Work out the finished part from the listing and answer in its coordinate system (mm). Round coordinates to 2 decimals unless told otherwise and drop trailing zeros. Order: outer loops, then holes, each group sorted by start corner. A loop starts at its lowest first (then second) coordinate and runs counter-clockwise, first axis right, second up. Notation, with made-up numbers: (42, 48) -> (46, 48) arc R16 ccw to (46, 72) -> close; hole circle Ø9 at (1, 41.25). An arc over 180 degrees is marked (long way). Use one line per item in the form item = value.
```python
from build123d import *

# Parameters (mm, degrees)
SKETCH_1_R          = 1.75
EXTRUDE_1_DEPTH     = 2
SKETCH_3_R          = 1.5
CUT_EXTRUDE_1_DEPTH = 10


with BuildPart() as part:
    # 草图1 → 凸台-拉伸1 (new body)
    with BuildSketch(Plane(origin=(0, 0, 0), x_dir=(1, 0, 0), z_dir=(0, 1, 0))):
        with BuildLine():
            Line((-44.248197972, 34.748679798), (44.751802028, 34.748679798))
            ThreePointArc((44.751802028, 34.748679798), (46.16601559, 34.16289336), (46.751802028, 32.748679798))
            Line((46.751802028, 32.748679798), (46.751802028, -32.251320202))
            ThreePointArc((46.751802028, -32.251320202), (46.16601559, -33.665533764), (44.751802028, -34.251320202))
            Line((44.751802028, -34.251320202), (-45.248197972, -34.251320202))
            ThreePointArc((-45.248197972, -34.251320202), (-46.662411535, -33.665533764), (-47.248197972, -32.251320202))
            Line((-47.248197972, -32.251320202), (-47.248197972, 31.748679798))
            ThreePointArc((-47.248197972, 31.748679798), (-46.369518316, 33.870000142), (-44.248197972, 34.748679798))
        make_face()
        with Locations(Location((-43.029034064, 30.65, 0), (0, 0, 270))):
            Circle(SKETCH_1_R, mode=Mode.SUBTRACT)
        with Locations(Location((43.468694969, 30.023204862, 0), (0, 0, 90))):
            Circle(SKETCH_1_R, mode=Mode.SUBTRACT)
        with Locations(Location((43.468694969, -30.023204862, 0), (0, 0, 270))):
            Circle(SKETCH_1_R, mode=Mode.SUBTRACT)
        with Locations(Location((-43.029034064, -30.65, 0), (0, 0, 90))):
            Circle(SKETCH_1_R, mode=Mode.SUBTRACT)
    extrude(amount=EXTRUDE_1_DEPTH)

    # 草图3 → 切除-拉伸1 (cut)
    with BuildSketch(Plane(origin=(0, 2, 0), x_dir=(1, 0, 0), z_dir=(0, 1, 0))):
        with Locations(Location((-40, -20, 0), (0, 0, 270))):
            Circle(SKETCH_3_R)
        with Locations(Location((40, -20, 0), (0, 0, 270))):
            Circle(SKETCH_3_R)
        with Locations(Location((40, 20, 0), (0, 0, 270))):
            Circle(SKETCH_3_R)
        with Locations(Location((-40, 20, 0), (0, 0, 270))):
            Circle(SKETCH_3_R)
    extrude(amount=-CUT_EXTRUDE_1_DEPTH, mode=Mode.SUBTRACT)


solid = part.part
```
Item 1: A flat-ended cylindrical pin translates along its axis: P1, Ø3, axis at x = -43.03, z = -30.65, coming from the -Y side. Find the tip coordinate at first contact, or state that the pin passes through.
Findings:
P1 = through
Item 2: Determine the mould class of faces 1 (the cylindrical face through (-46.65, 0.99, 33.68)), 2 (the cylindrical face through (-40.9, 1, 18.8)), 3 (the cylindrical face through (46.18, 0.99, 33.65)) for opening direction X: released by +X, released by -X, zero draft, split by the parting line, or undercut.
Findings:
face_1 = released by -X
face_2 = undercut
face_3 = released by +X
Item 3: The part is cut by section B-B, the plane z = 20. Give the vertices of the cut face in (x, y), and give its area (3 significant figures).
Findings:
outline = (-47.25, 0) -> (-41.5, 0) -> (-41.5, 2) -> (-47.25, 2) -> close; (-38.5, 0) -> (38.5, 0) -> (38.5, 2) -> (-38.5, 2) -> close; (41.5, 0) -> (46.75, 0) -> (46.75, 2) -> (41.5, 2) -> close
area = 176 mm^2
Item 4: The part is cut by section A-A, the plane x = 40. Give the vertices of the cut face in (y, z), and give its area (3 significant figures).
Findings:
outline = (0, -34.75) -> (2, -34.75) -> (2, -21.5) -> (0, -21.5) -> close; (0, -18.5) -> (2, -18.5) -> (2, 18.5) -> (0, 18.5) -> close; (0, 21.5) -> (2, 21.5) -> (2, 34.25) -> (0, 34.25) -> close
area = 126 mm^2
Item 5: Consider line 1 along X through (y, z) = (0.8, -20); line 2 along X through (y, z) = (1.35, -30.65). Determine where each line is inside the solid, lowest interval first.
Findings:
line_1 = -47.25 to -41.5, -38.5 to 38.5, 41.5 to 46.75
line_2 = -47.25 to -44.78, -41.28 to 41.83, 45.1 to 46.75
